Work out the finished part from the listing and answer in its coordinate system (mm). Face numbers are marked on the shaded views. A direction names the side the tool comes from. Round coordinates to 2 decimals unless told otherwise and drop trailing zeros. Order: outer loops, then holes, each group sorted by start corner. A loop starts at its lowest first (then second) coordinate and runs counter-clockwise, first axis right, second up. Notation, with made-up numbers: (80, 72.25) - (132, 72.25) arc R25 ccw to (132, 111.25) - close; hole circle Ø1 at (57, -17). An arc over 180 degrees is marked (long way). Put each result on its own line as item: value.
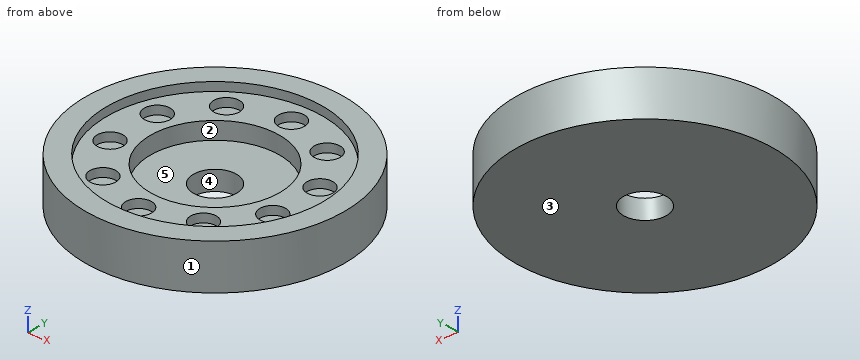
```python
from build123d import *

# Parameters (mm, degrees)
SKETCH2_R           = 381
BOSS_EXTRUDE1_DEPTH = 133.35
SKETCH3_R           = 317.5
CUT_EXTRUDE1_DEPTH  = 25.4
SKETCH4_R           = 38.1
CUT_EXTRUDE2_DEPTH  = 25.4
SKETCH5_R           = 190.5
CUT_EXTRUDE3_DEPTH  = 50.8
SKETCH6_R           = 63.5
CUT_EXTRUDE4_DEPTH  = 545.176846255


with BuildPart() as part:
    # Sketch2 → Boss-Extrude1 (new body)
    with BuildSketch(Plane.XY):
        Circle(SKETCH2_R)
    extrude(amount=BOSS_EXTRUDE1_DEPTH)

    # Sketch3 → Cut-Extrude1 (cut)
    with BuildSketch(Plane.XY.offset(133.35)):
        Circle(SKETCH3_R)
    extrude(amount=-CUT_EXTRUDE1_DEPTH, mode=Mode.SUBTRACT)

    # Sketch4 → Cut-Extrude2 (cut)
    with BuildSketch(Plane.XY.offset(107.95)):
        with Locations((0, 254)):
            Circle(SKETCH4_R)
        with Locations((149.297454082, 205.490316571)):
            Circle(SKETCH4_R)
        with Locations((241.568355139, 78.490316571)):
            Circle(SKETCH4_R)
        with Locations((241.568355139, -78.490316571)):
            Circle(SKETCH4_R)
        with Locations((149.297454082, -205.490316571)):
            Circle(SKETCH4_R)
        with Locations((0, -254)):
            Circle(SKETCH4_R)
        with Locations((-149.297454082, -205.490316571)):
            Circle(SKETCH4_R)
        with Locations((-241.568355139, -78.490316571)):
            Circle(SKETCH4_R)
        with Locations((-241.568355139, 78.490316571)):
            Circle(SKETCH4_R)
        with Locations((-149.297454082, 205.490316571)):
            Circle(SKETCH4_R)
    extrude(amount=-CUT_EXTRUDE2_DEPTH, mode=Mode.SUBTRACT)

    # Sketch5 → Cut-Extrude3 (cut)
    with BuildSketch(Plane.XY.offset(107.95)):
        Circle(SKETCH5_R)
    extrude(amount=-CUT_EXTRUDE3_DEPTH, mode=Mode.SUBTRACT)

    # Sketch6 → Cut-Extrude4 (cut, through all)
    with BuildSketch(Plane.XY.offset(57.15)):
        Circle(SKETCH6_R)
    extrude(amount=-CUT_EXTRUDE4_DEPTH, mode=Mode.SUBTRACT)


solid = part.part
```
1) For a pull along X with two mould halves and no side action, classify the marked faces 1, 2 and 3 as pulls with the +X half, pulls with the -X half, needs draft (parallel to the pull), parting line crosses it, or undercut.
Findings below:
face 1: parting line crosses it
face 2: undercut
face 3: needs draft
2) Given pin 1 Ø23 at (x, y) = (250.5, 94.5) entering from +Z; pin 2 Ø1 at (y, z) = (-100.5, 104.5) entering from -X; pin 3 Ø8 at (x, y) = (4, -197) entering from -Z; pin 4 Ø2 at (x, z) = (-183.5, 66) entering from -Y, each flat-ended and moving along its own axis, determine where each tip first touches the part or whether it passes through.
Findings below:
pin 1: stops at z = 82.55
pin 2: stops at x = -367.64
pin 3: stops at z = 0
pin 4: stops at y = -334.45
3) For the marked faces 4 and 5, determine the directions among +Z, -Z, +X, -X, +Y, -Y from which every point of the face is accessible in a straight line to the end or side of a thin tool.
Findings below:
face 4: +Z, -Z
face 5: +Z
4) A cutting plane is placed at D-D on y = 254. Write down the section's boundary in (x, z), then the cut area to 3 significant figures.
Findings below:
outline: (-283.98, 0) - (283.98, 0) - (283.98, 133.35) - (190.5, 133.35) - (190.5, 107.95) - (38.1, 107.95) - (38.1, 82.55) - (-38.1, 82.55) - (-38.1, 107.95) - (-190.5, 107.95) - (-190.5, 133.35) - (-283.98, 133.35) - close
area: 64,100 mm2
5) A cutting plane is placed at B-B on y = 0. Write down the section's boundary in (x, z), then the cut area to 3 significant figures.
Findings below:
outline: (-381, 0) - (-63.5, 0) - (-63.5, 57.15) - (-190.5, 57.15) - (-190.5, 107.95) - (-317.5, 107.95) - (-317.5, 133.35) - (-381, 133.35) - close; (63.5, 0) - (381, 0) - (381, 133.35) - (317.5, 133.35) - (317.5, 107.95) - (190.5, 107.95) - (190.5, 57.15) - (63.5, 57.15) - close
area: 58,900 mm2
6) Straight lines are drawn through the part: L1, parallel to Y at x = 0, z = 101; L2, parallel to X at y = 93, z = 88; L3, parallel to Y at x = 208, z = 106. For each, find the intervals that lie inside material, in ascending order. Write a range as from..to.
Findings below:
L1: y = -381..-292.1, -215.9..-190.5, 190.5..215.9, 292.1..381
L2: x = -369.48..-276.8, -206.34..-166.26, 166.26..206.34, 276.8..369.48
L3: y = -319.21..-96.51, -60.47..60.47, 96.51..319.21
7) A cutting plane is placed at A-A on x = 0. Write down the section's boundary in (y, z).
Findings below:
outline: (-381, 0) - (-63.5, 0) - (-63.5, 57.15) - (-190.5, 57.15) - (-190.5, 107.95) - (-215.9, 107.95) - (-215.9, 82.55) - (-292.1, 82.55) - (-292.1, 107.95) - (-317.5, 107.95) - (-317.5, 133.35) - (-381, 133.35) - close; (63.5, 0) - (381, 0) - (381, 133.35) - (317.5, 133.35) - (317.5, 107.95) - (292.1, 107.95) - (292.1, 82.55) - (215.9, 82.55) - (215.9, 107.95) - (190.5, 107.95) - (190.5, 57.15) - (63.5, 57.15) - close
8) A cutting plane is placed at C-C on z = 99. Give the number of separate pieces and of enclosed holes in the cut face, then the cut area to 3 significant figures.
Findings below:
separate pieces: 1
enclosed holes: 11
area: 296,000 mm2
